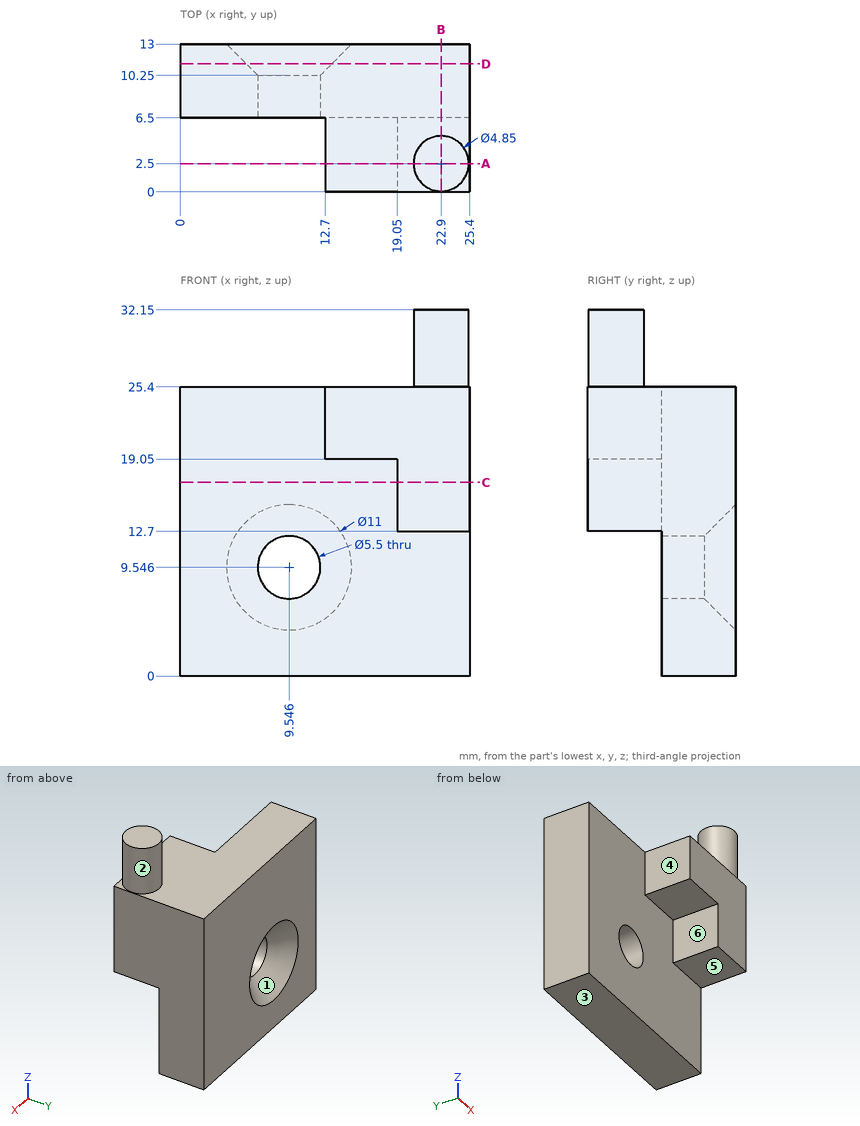
Design review of the part shown in the three views and the two pictorial views. Dimensions are in mm from the part's minimum x, y and z. A direction names the side the tool comes from. Round coordinates to 2 decimals unless told otherwise and drop trailing zeros. Loops run counter-clockwise (first coordinate to the right, second up) from the corner with the lowest first, then second, coordinate; pieces in that order, holes last.
Q1. Mouldability with a two-part tool opening along X and no side actions: class the marked faces 1, 2 and 3 as +X half, -X half, draft (parallel to the pull), parting line (faces both ways), or undercut.
Result sheet:
face 1: undercut
face 2: parting line
face 3: draft
Q2. Add section A-A on y = 2.5. Write out the cut boundary in (x, z) (3 decimals).
Result sheet:
outline: (12.7, 19.05) - (19.05, 19.05) - (19.05, 12.7) - (25.4, 12.7) - (25.4, 25.4) - (25.325, 25.4) - (25.325, 32.15) - (20.475, 32.15) - (20.475, 25.4) - (12.7, 25.4) - close
Q3. To check wall thickness, follow line 1 along Y through (x, z) = (4.75, 25); line 2 along Z through (x, y) = (10, 10.25); line 3 along Z through (x, y) = (1.75, 12). State the ranges of each line that lie inside material, in increasing order.
Result sheet:
line 1: y = 6.5 to 13
line 2: z = 0 to 6.83, 12.26 to 25.4
line 3: z = 0 to 25.4
Q4. Add section C-C on z = 17. Write out the cut boundary in (x, y).
Result sheet:
outline: (0, 6.5) - (19.05, 6.5) - (19.05, 0) - (25.4, 0) - (25.4, 13) - (0, 13) - close
Q5. Machinability: for the marked faces 4, 5 and 6, which of the approach directions +Z, -Z, +X, -X, +Y, -Y give a long, thin tool a straight path to every point of the face, cutting with its end or side? Answer none if there is none.
Result sheet:
face 4: +Z, -Z, -X, -Y
face 5: -Z, +X, -X, -Y
face 6: -Z, -X, -Y
Q6. Add section B-B on x = 22.9. Write out the cut boundary in (y, z) (3 decimals).
Result sheet:
outline: (0, 12.7) - (6.5, 12.7) - (6.5, 0) - (13, 0) - (13, 25.4) - (4.925, 25.4) - (4.925, 32.15) - (0.075, 32.15) - (0.075, 25.4) - (0, 25.4) - close
Q7. Insertion check: pin 1 Ø7 at (y, z) = (4.5, 21.5) entering from -X; pin 2 Ø10 at (x, z) = (3, 17) entering from -Y; pin 3 Ø5 at (x, y) = (22, 3.5) entering from -Z; pin 4 Ø7 at (x, z) = (9.55, 9.55) entering from +Y. Each pin has a flat end and moves straight along its axis. Give the tip position at first contact, or say it passes through.
Result sheet:
pin 1: stops at x = 0
pin 2: stops at y = 6.5
pin 3: stops at z = 12.7
pin 4: stops at y = 11.01
Q8. Add section D-D on y = 11.25. Write out the cut boundary in (x, z).
Result sheet:
outline: (0, 0) - (25.4, 0) - (25.4, 25.4) - (0, 25.4) - close; hole circle Ø7.5 at (9.55, 9.55)
